Model file for the job. Use its own axes, mm. Face numbers are marked on the shaded views. A direction names the side the tool comes from. Coordinates: 2 decimals unless noted, no trailing zeros. Write each loop counter-clockwise with the first axis right and the second up, starting at its lowest first coordinate (ties: lowest second). Pieces come first, ordered by that corner, then holes. Notation, with made-up numbers: (23, -31) - (64, -31) arc R22 cw to (64, -21) - close; hole circle Ø8 at (-24.75, 72.25). An arc over 180 degrees is marked (long way). Put each result on its own line as item: value. Start each with the question number.
1. Saw through at D-D, the plane y = 3.5. Write the cut outline in (x, z).
2. Which spindle directions (+Z, -Z, +X, -X, +Y, -Y) get a long thin tool onto all of the face, cutting with end or side? Do the marked faces 4 and 5. Say none if no direction does.
3. Saw through at B-B, the plane z = 1.25. Write the cut outline in (x, y).
4. Saw through at C-C, the plane x = 0. Write the cut outline in (y, z), plus the area to 3 significant figures.
5. Drill centre lines: L1, parallel to X at y = 4.2, z = 14; L2, parallel to Z at x = 3.5, y = 9; L3, parallel to Z at x = 0, y = 5.6. Where is each one in solid material? Low to high. Write a range as from..to.
6. Drop flat-ended pins along their axis: P1, Ø2, axis at x = -1.5, z = -1, coming from the +Y side; P2, Ø3, axis at x = 3.5, y = 4.5, coming from the -Z side; P3, Ø2, axis at x = 0.5, z = -2.5, coming from the -Y side. Give the stop position or say it passes through.
7. Saw through at A-A, the plane y = 9. Write the cut outline in (x, z), plus the area to 3 significant figures.
8. Pull direction X, two halves, no side cores. Call the marked faces 1, 2 and 3: released by +X, released by -X, zero draft, split by the parting line, or undercut.
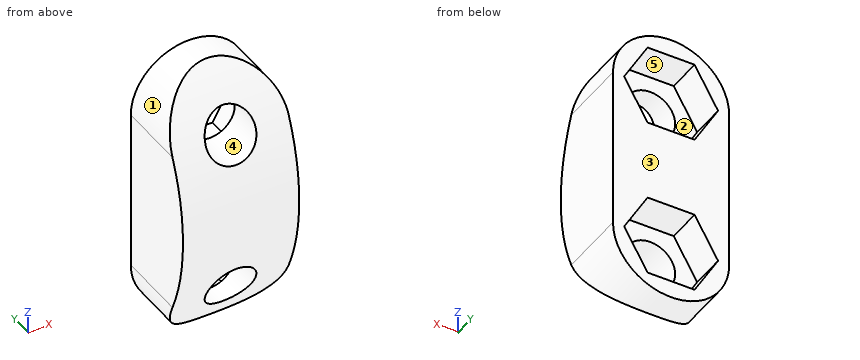
Autodesk Inventor part; units mm, degrees
ref_plane "YZ Plane" through (0, 0, 0) normal (1, 0, 0) x (0, 1, 0)
ref_plane "XZ Plane" through (0, 0, 0) normal (0, 1, 0) x (-1, 0, 0)
ref_plane "XY Plane" through (0, 0, 0) normal (0, 0, 1) x (1, 0, 0)
sketch "Sketch1" plane through (0, 0, 0) normal (0, 1, 0) x (-1, 0, 0)
  arc A0 (-5, 0) -> (5, 0) centre (0, 0) ccw
  circle A1 centre (0, 0) radius 2.15
  arc A2 (5, 14) -> (-5, 14) centre (0, 14) ccw
  circle A3 centre (0, 14) radius 2.15
  line L0 (-5, 0) -> (-5, 14)
  line L1 (5, 0) -> (5, 14)
  line L2 (0, 0) -> (0, 2.15)
  line L3 (0, 9) -> (0, 14)
  dimension "d1" = 4.3
  dimension "d0" = 10
  dimension "d9" = 14
  dimension "d10" = 10
  dimension "d11" = 4.3
extrude "Extrusion1" add sketch "Sketch1" along normal blind 10
sketch "Sketch2" plane through (0, 10, 0) normal (0, 1, 0) x (-1, 0, 0)
  line L0 (2.0207, 3.5) -> (4.0415, 0)
  line L1 (4.0415, 0) -> (2.0207, -3.5)
  line L2 (2.0207, -3.5) -> (-2.0207, -3.5)
  line L3 (-2.0207, -3.5) -> (-4.0415, 0)
  line L4 (-4.0415, 0) -> (-2.0207, 3.5)
  line L5 (-2.0207, 3.5) -> (2.0207, 3.5)
  circle A0 centre (0, 14) radius 2.15
  line L6 (-4.0415, 14) -> (-2.0207, 17.5)
  line L7 (-2.0207, 17.5) -> (2.0207, 17.5)
  line L8 (2.0207, 17.5) -> (4.0415, 14)
  line L9 (4.0415, 14) -> (2.0207, 10.5)
  line L10 (2.0207, 10.5) -> (-2.0207, 10.5)
  line L11 (-2.0207, 10.5) -> (-4.0415, 14)
  point P0 (0, 0)
  point P1 (0, 0)
  dimension "d4" = 7
  dimension "d15" = 7
extrude "Extrusion2" cut sketch "Sketch2" against normal blind 3
sketch "Sketch3" plane through (0, 0, 0) normal (1, 0, 0) x (0, 1, 0)
  line L0 (0, 0) -> (0, 7)
  line L1 (0, 2.15) -> (0, -2.15)
  line L2 (0, 7) -> (19.5, 7)
  circle A0 centre (19.5, 7) radius 17
  line L3 (7, -2.15) -> (7, 2.15)
  line L4 (7, 0) -> (7, 3.5)
  line L5 (7, -3.5) -> (7, 0)
  line L6 (7, 0) -> (7, -3.5)
  line L7 (7, 3.5) -> (7, 0)
  circle A1 centre (19.5, 7) radius 30.634
  dimension "d7" = 7
  dimension "d8" = 19.5
  dimension "d12" = 34
extrude "Extrusion3" cut sketch "Sketch3" along normal through all both and the other way through all
equation "\"d15\" = d4"
properties part number "Spacer_Collective_Base_NutM4"
Final values:
1. outline: (-5, 1.26) - (-1.75, 1.26) arc R2.15 cw to (1.75, 1.26) - (5, 1.26) - (5, 12.74) - (1.75, 12.74) arc R2.15 cw to (-1.75, 12.74) - (-5, 12.74) - close
2. face 4: +Y, -Y
2. face 5: +Y
3. outline: (-5, 3.5) - (-1.75, 3.5) - (-1.75, 7) - (-3.32, 7) - (-3.32, 10) - (-5, 10) - close; (1.75, 3.5) - (5, 3.5) - (5, 10) - (3.32, 10) - (3.32, 7) - (1.75, 7) - close
4. outline: (3.21, 2.15) - (7, 2.15) - (7, 3.5) - (10, 3.5) - (10, 10.5) - (7, 10.5) - (7, 11.85) - (3.21, 11.85) arc R17 ccw to start; (5.17, -2.15) arc R17 ccw to (7.46, -5) - (10, -5) - (10, -3.5) - (7, -3.5) - (7, -2.15) - close; (5.17, 16.15) - (7, 16.15) - (7, 17.5) - (10, 17.5) - (10, 19) - (7.46, 19) arc R17 ccw to start
4. area: 75.8 mm²
5. L1: x = -5..-2.15, 2.15..5
5. L2: z = -3.57..-0.94, 0.94..13.06, 14.94..17.57
5. L3: z = -2.79..-2.15, 2.15..11.85, 16.15..16.79
6. P1: stops at y = 7
6. P2: stops at z = -3.33
6. P3: stops at y = 4.95
7. outline: (-5, 0) arc R5 ccw to (5, 0) - (5, 14) arc R5 ccw to (-5, 14) - close; hole (-4.04, 0) - (-2.02, -3.5) - (2.02, -3.5) - (4.04, 0) - (2.02, 3.5) - (-2.02, 3.5) - close; hole (-4.04, 14) - (-2.02, 10.5) - (2.02, 10.5) - (4.04, 14) - (2.02, 17.5) - (-2.02, 17.5) - close
7. area: 134 mm²
8. face 1: split by the parting line
8. face 2: undercut
8. face 3: zero draft
